from build123d import *

# Parameters (mm, degrees)
F0_W     = 36
F0_H     = 79
F0_W_2   = 16
F0_H_2   = 75
F0_R     = 3
F1_DEPTH = 2
F2_DEPTH = 25
F0_R_2   = 1.5
F3_DEPTH = 3
F4_R     = 1.99999
F5_W     = 15
F5_H     = 5
F6_DEPTH = 100


# Not quite as in the source:
# - a fillet or chamfer is up to 0.001 mm smaller than in the source, because OpenCascade refuses the exact size


with BuildPart() as f1:
    # F0 (on Top) → F1 (new body)
    with BuildSketch(Plane.XY):
        Rectangle(F0_W, F0_H)
        Polygon((0, 37.5), (16, 37.5), (16, -37.5), (0, -37.5), (-16, -37.5), (-16, 37.5), align=None, mode=Mode.SUBTRACT)
        with Locations((8, 0)):
            Rectangle(F0_W_2, F0_H_2)
        with Locations((-8, 0)):
            Rectangle(F0_W_2, F0_H_2)
        with Locations((-10, -25)):
            Circle(F0_R, mode=Mode.SUBTRACT)
        with Locations((-10, 25)):
            Circle(F0_R, mode=Mode.SUBTRACT)
    extrude(amount=F1_DEPTH)

    # F0 (on Top) → F2 (join)
    with BuildSketch(Plane.XY):
        Rectangle(F0_W, F0_H)
        Polygon((0, 37.5), (16, 37.5), (16, -37.5), (0, -37.5), (-16, -37.5), (-16, 37.5), align=None, mode=Mode.SUBTRACT)
    extrude(amount=F2_DEPTH)

    # F0 (on Top) → F3 (join)
    with BuildSketch(Plane.XY):
        with Locations((-8, 0)):
            Rectangle(F0_W_2, F0_H_2)
        with Locations((-10, -25)):
            Circle(F0_R, mode=Mode.SUBTRACT)
        with Locations((-10, 25)):
            Circle(F0_R, mode=Mode.SUBTRACT)
        with Locations((-10, 25)):
            Circle(F0_R)
        with Locations((-10, 25)):
            Circle(F0_R_2, mode=Mode.SUBTRACT)
        with Locations((-10, -25)):
            Circle(F0_R)
        with Locations((-10, -25)):
            Circle(F0_R_2, mode=Mode.SUBTRACT)
    extrude(amount=-F3_DEPTH)

    # F4 (radius 2 in the source; OpenCascade refuses exactly that, so slightly less here)
    f4_edges = [f1.edges().sort_by_distance(p)[0] for p in [
        (-18, 0, 0),
        (0, -39.5, 0),
        (0, 39.5, 0),
        (18, 0, 0),
        (18, 39.5, 12.5),
        (-18, 39.5, 12.5),
        (-18, -39.5, 12.5),
        (18, -39.5, 12.5),
    ]]
    fillet(f4_edges, radius=F4_R)

    # F5 (on face) → F6 (cut)
    with BuildSketch(Plane.XZ.offset(39.5)):
        with Locations((0, 13.0054904148)):
            Rectangle(F5_W, F5_H)
    extrude(amount=-F6_DEPTH, mode=Mode.SUBTRACT)


solid = f1.part
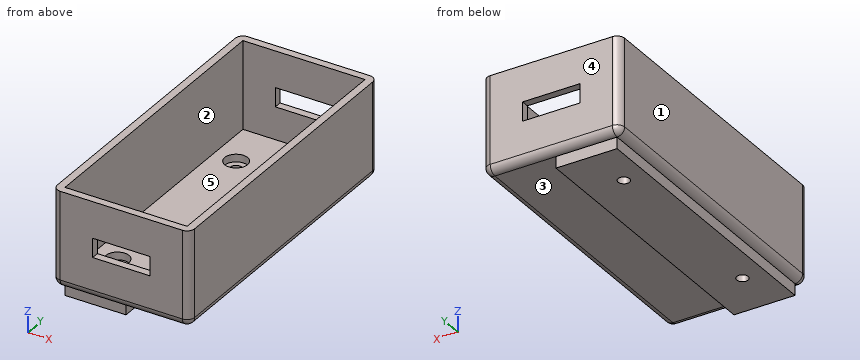
Read the model definition and answer for the solid it produces. Units are mm, in the model's axes. Face numbers are marked on the shaded views. A direction names the side the tool comes from. Coordinates: 2 decimals unless noted, no trailing zeros. Loops run counter-clockwise (first coordinate to the right, second up) from the corner with the lowest first, then second, coordinate; pieces in that order, holes last. Notation, with made-up numbers: (-38, 4.25) -> (17, 4.25) arc R25 ccw to (17, 21.25) -> close; hole circle Ø4 at (-18, 5). An arc over 180 degrees is marked (long way). Answer in a Markdown table with one row per item.
Item 1: For the marked faces 1 and 2, determine the directions among +Z, -Z, +X, -X, +Y, -Y from which every point of the face is accessible in a straight line to the end or side of a thin tool.
Returned:
| item | result |
|---|---|
| face 1 | +Z, -Z, -X, +Y, -Y |
| face 2 | +Z |
Item 2: A cutting plane is placed at B-B on x = -10. Give the number of separate pieces and of enclosed holes in the cut face, plus the area to 3 significant figures.
Returned:
| item | result |
|---|---|
| separate pieces | 3 |
| enclosed holes | 0 |
| area | 431 mm^2 |
Item 3: A cutting plane is placed at C-C on z = 8.25. Determine the outline of the cut face in (x, y).
Returned:
| item | result |
|---|---|
| outline | (-18, -37.5) arc R2 ccw to (-16, -39.5) -> (16, -39.5) arc R2 ccw to (18, -37.5) -> (18, 37.5) arc R2 ccw to (16, 39.5) -> (-16, 39.5) arc R2 ccw to (-18, 37.5) -> close; hole (-16, -37.5) -> (16, -37.5) -> (16, 37.5) -> (-16, 37.5) -> close |
Item 4: Straight lines are drawn through the part: line 1 along Y through (x, z) = (-10, -2.1); line 2 along X through (y, z) = (-34, 18.25); line 3 along Y through (x, z) = (13.5, 3.25). For each, find the intervals that lie inside material, in ascending order. Write a range as [from, to].
Returned:
| item | result |
|---|---|
| line 1 | y = [-37.5, -26.5], [-23.5, 23.5], [26.5, 37.5] |
| line 2 | x = [-18, -16], [16, 18] |
| line 3 | y = [-39.5, -37.5], [37.5, 39.5] |
Item 5: Each of these flat-tipped pins is pushed along its axis until it touches: P1, Ø3.5, axis at x = -4, z = -1.5, coming from the -Y side; P2, Ø1, axis at y = 38.5, z = 12, coming from the +X side; P3, Ø6, axis at x = -8.5, y = -7.5, coming from the +Z side. Where does it stop, or does it pass through?
Returned:
| item | result |
|---|---|
| P1 | stops at y = -38.47 |
| P2 | stops at x = 17.94 |
| P3 | stops at z = 2 |
Item 6: A cutting plane is placed at D-D on x = 13.5. Determine the outline of the cut face in (y, z).
Returned:
| item | result |
|---|---|
| outline | (-39.5, 2) arc R2 ccw to (-37.5, 0) -> (37.5, 0) arc R2 ccw to (39.5, 2) -> (39.5, 25) -> (37.5, 25) -> (37.5, 2) -> (-37.5, 2) -> (-37.5, 25) -> (-39.5, 25) -> close |
Item 7: For a pull along Y with two mould halves and no side action, classify the marked faces 3, 4 and 5 as released by +Y, released by -Y, zero draft, split by the parting line, or undercut.
Returned:
| item | result |
|---|---|
| face 3 | zero draft |
| face 4 | released by +Y |
| face 5 | undercut |
